CAD build for the part. Positions are in the model's coordinates, mm. A direction names the side the tool comes from. Coordinates: 2 decimals unless noted, no trailing zeros. Loops run counter-clockwise (first coordinate to the right, second up) from the corner with the lowest first, then second, coordinate; pieces in that order, holes last. Notation, with made-up numbers: (78, 65.5) -> (105, 65.5) arc R13 ccw to (105, 79.5) -> close; hole circle Ø1 at (21, 59). An arc over 180 degrees is marked (long way). Write item = value, one per line. Start each with the question number.
(1) Tool access for faces 4 (the face through (14, 3.47, -3)), 5 (the face through (-4, 1.32, 1)), 6 (the face through (14, 2.92, 2)): list every direction of +Z, -Z, +X, -X, +Y, -Y with a clear straight run to the whole face (end or side of a thin tool).
(2) Drill centre lines: line 1 (Z direction, x = 7.75, y = 3.3); line 2 (Y direction, x = 10, z = -3.25); line 3 (Y direction, x = -4, z = -2.25). Where is each one in solid material? Low to high. Write a range as from..to.
(3) Pull direction X, two halves, no side cores. Call faces 1 (the face through (14, 2.92, -3)), 2 (the face through (-3.512, 0.651, -0.591)), 3 (the face through (-1.36, 3.08, -0.44)): +X half, -X half, draft (parallel to the pull), parting line (faces both ways), or undercut.
(4) Band-saw the part on C-C (z = -4.75). Write the cut outline in (x, y) (3 decimals), and give its area (3 significant figures).
(5) Band-saw the part on B-B (x = 11.5). Write the cut outline in (y, z).
(6) Flat gauge pins, fed straight in: P1, Ø3, axis at x = 15.5, z = -1.5, coming from the -Y side; P2, Ø1, axis at x = 15, y = 3.5, coming from the -Z side; P3, Ø2, axis at x = 9, y = 3, coming from the +Z side. Where does each tip first touch, or does it go through?
(7) Band-saw the part on A-A (z = 1). Write the cut outline in (x, y) (3 decimals).
(8) Band-saw the part on D-D (x = -4.5). Write the cut outline in (y, z).
Autodesk Inventor part; units mm, degrees
ref_plane "YZ Plane" through (0, 0, 0) normal (1, 0, 0) x (0, 1, 0)
ref_plane "XZ Plane" through (0, 0, 0) normal (0, 1, 0) x (-1, 0, 0)
ref_plane "XY Plane" through (0, 0, 0) normal (0, 0, 1) x (1, 0, 0)
sketch "Sketch1" plane through (0, 0, 0) normal (0, 1, 0) x (-1, 0, 0)
  line L0 (-7.0894, 4.7564) -> (8.1506, 4.7564)
  line L1 (8.1506, 4.7564) -> (8.1506, -5.7836)
  line L2 (8.1506, -5.7836) -> (-7.0894, -5.7836)
  line L3 (-7.0894, -5.7836) -> (-7.0894, 4.7564)
  circle A0 centre (5.2806, -0.5136) radius 1.77
  point P0 (0, 0)
  dimension "d0" = 10.54
  dimension "d1" = 15.24
  dimension "d2" = 3.54
  dimension "d3" = 2.87
  dimension "d4" = 5.27
extrude "Extrusion1" add sketch "Sketch1" along normal blind 1.32
sketch "Sketch2" plane through (0, 1.32, 0) normal (0, 1, 0) x (1, 0, 0)
  line L0 (7.0894, 5.7836) -> (-8.1506, 5.7836)
  line L1 (-2.0506, 5.7836) -> (7.0894, 5.7836)
  line L2 (7.0894, 5.7836) -> (7.0894, -4.7564)
  line L3 (7.0894, -4.7564) -> (-2.0506, -4.7564)
  line L4 (-2.0506, -4.7564) -> (-2.0506, 5.7836)
  point P0 (0, 0)
  dimension "d7" = 9.14
extrude "Extrusion2" add sketch "Sketch2" along normal blind 3.37
chamfer "Chamfer1" distance 1.4 distance2 3.175 1 edges at (-2.0506, 4.69, -0.5136) measured on face at (0.996, 4.69, -2.2703)
chamfer "Chamfer2" distance 0.5 distance2 3.175 1 edges at (3.2194, 4.69, -5.7836) measured on face at (1.9294, 4.69, -2.2703)
chamfer "Chamfer3" distance 0.5 distance2 3.175 1 edges at (3.2194, 4.69, 4.7564) measured on face at (1.9294, 4.69, -1.9369)
sketch "Sketch4" plane through (7.0894, 0, 4.7564) normal (1, 0, 0) x (0, 0, -1)
  line L0 (0, 0) -> (0, 1.515)
  line L1 (10.54, 0) -> (0, 0)
  line L2 (2.03, 3.47) -> (8.51, 3.47)
  line L3 (8.51, 3.47) -> (8.51, 2.92)
  line L4 (8.51, 2.92) -> (2.03, 2.92)
  line L5 (2.03, 2.92) -> (2.03, 3.47)
  line L6 (3.43, 3.47) -> (3.43, 2.92)
  line L7 (4.57, 3.47) -> (4.57, 2.92)
  line L8 (5.97, 3.47) -> (5.97, 2.92)
  line L9 (7.11, 3.47) -> (7.11, 2.92)
  point P0 (4.7564, 0)
  dimension "d19" = 0.55
  dimension "d20" = 2.92
  dimension "d21" = 6.48
  dimension "d22" = 1.4
  dimension "d23" = 1.4
  dimension "d24" = 1.4
  dimension "d25" = 2.54
  dimension "d26" = 4.57
extrude "Extrusion3" add sketch "Sketch4" along normal blind 14 contours L2 L6 L4 L5 | L2 L8 L4 L7 | L2 L3 L4 L9
properties part number "MOSFET"
Findings below:
q1.face_4 = +Z, -Z, +X, +Y
q1.face_5 = +Z, -Z, -X, +Y
q1.face_6 = +Z, -Z, +X, -Y
q2.line_1 = -3.75..-2.35, -1.21..0.19, 1.33..2.73
q2.line_2 = 2.92..3.47
q2.line_3 = 0..1.32
q3.face_1 = draft
q3.face_2 = undercut
q3.face_3 = -X half
q4.outline = (-8.151, 0) -> (7.089, 0) -> (7.089, 4.69) -> (-0.651, 4.69) -> (-2.051, 1.515) -> (-2.051, 1.32) -> (-8.151, 1.32) -> close
q4.area = 48.7 mm²
q5.outline = (2.92, -3.75) -> (3.47, -3.75) -> (3.47, -2.35) -> (2.92, -2.35) -> close; (2.92, -1.21) -> (3.47, -1.21) -> (3.47, 0.19) -> (2.92, 0.19) -> close; (2.92, 1.33) -> (3.47, 1.33) -> (3.47, 2.73) -> (2.92, 2.73) -> close
q6.P1 = 2.92
q6.P2 = -3.75
q6.P3 = 2.73
q7.outline = (-8.151, 0) -> (-6.198, 0) -> (-6.198, 1.32) -> (-8.151, 1.32) -> close; (-4.363, 0) -> (7.089, 0) -> (7.089, 4.69) -> (-0.651, 4.69) -> (-2.051, 1.515) -> (-2.051, 1.32) -> (-4.363, 1.32) -> close
q8.outline = (0, -5.78) -> (1.32, -5.78) -> (1.32, -2.1) -> (0, -2.1) -> close; (0, 1.07) -> (1.32, 1.07) -> (1.32, 4.76) -> (0, 4.76) -> close
